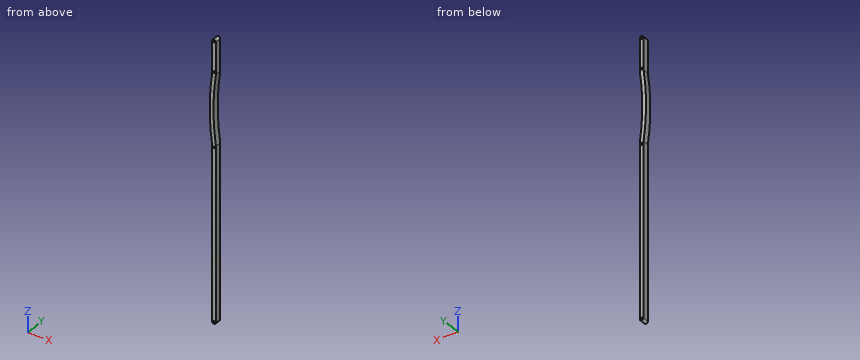
Autodesk Inventor part; units mm, degrees
ref_plane "YZ Plane" through (0, 0, 0) normal (1, 0, 0) x (0, 1, 0)
ref_plane "XZ Plane" through (0, 0, 0) normal (0, 1, 0) x (-1, 0, 0)
ref_plane "XY Plane" through (0, 0, 0) normal (0, 0, 1) x (1, 0, 0)
sketch "Sketch1" plane through (0, 0, 0) normal (0, 1, 0) x (-1, 0, 0)
  line L0 (0, 0) -> (0, -441.93) construction
  line L1 (-3, 0) -> (-3, -441.93)
  line L2 (3, -441.93) -> (3, 0)
  arc A0 (3, 0) -> (-3, 0) centre (0, 0) ccw
  arc A1 (-3, -441.93) -> (3, -441.93) centre (0, -441.93) ccw
  circle A2 centre (0, 0) radius 1.5
  circle A3 centre (0, -441.93) radius 1.5
  circle A4 centre (0, -48.203) radius 1.5
  circle A5 centre (0, -166.766) radius 1.5
  arc A6 (-3, -163.766) -> (-3, -51.203) centre (-399.0207, -107.4845) ccw
  arc A7 (3, -163.766) -> (3, -51.203) centre (-393.0207, -107.4845) ccw
  point P0 (0, -220.965)
  dimension "d0" = 6
  dimension "d1" = 441.93
  dimension "d2" = 3
  dimension "d3" = 3
  dimension "d20" = 3
  dimension "d21" = 48.203
  dimension "d22" = 3
  dimension "d23" = 166.766
  dimension "d24" = 400
  dimension "d25" = 400
  dimension "d26" = 3
  dimension "d28" = 3
extrude "Extrusion1" add sketch "Sketch1" along normal blind 10 contours A0 L2 A1 L1 A6 | A7 L2
sketch "Sketch2" plane through (0, 10, 0) normal (0, 1, 0) x (1, 0, 0)
  line L0 (3, 0) -> (3, 51.203)
  arc A0 (3, 163.766) -> (3, 51.203) centre (399.0207, 107.4845) ccw
  line L1 (3, 163.766) -> (3, 441.93)
  arc A1 (3, 441.93) -> (-3, 441.93) centre (0, 441.93) ccw
  line L2 (-3, 441.93) -> (-3, 163.766)
  arc A2 (-3, 163.766) -> (-3, 51.203) centre (393.0207, 107.4845) ccw
  line L3 (-3, 51.203) -> (-3, 0)
  arc A3 (-3, 0) -> (3, 0) centre (0, 0) ccw
  circle A4 centre (0, 0) radius 1.5
  circle A5 centre (0, 441.93) radius 1.5
  circle A6 centre (0, 166.766) radius 1.5
  circle A7 centre (0, 48.203) radius 1.5
  line L4 (-3, 258.3394) -> (0, 251.9059)
  line L5 (0, 251.9059) -> (3, 258.3394)
  dimension "d29" = 25
  dimension "d30" = 25
extrude "Extrusion2" [suppressed]
Design review of the part built by this model. Coordinates are the model's own, in mm. Give positions to 0.01 mm unless a question says otherwise; leave off trailing zeros. Order: outer loops, then holes, each group sorted by start corner. A loop starts at its lowest first (then second) coordinate and runs counter-clockwise, first axis right, second up. Notation, with made-up numbers: (-7.5, 35) -> (44.5, 35) arc R25 cw to (44.5, 48) -> close; hole circle Ø1 at (50.25, 15.25). An arc over 180 degrees is marked (long way). Write item = value, one per line. Start each with the question number.
(1) To check wall thickness, follow line 1 along X through (y, z) = (9, -321); line 2 along X through (y, z) = (5.75, -441.93); line 3 along Z through (x, y) = (-2.25, 3.5). State the ranges of each line that lie inside material, in increasing order.
(2) We need section A-A on y = 6.25. Write out the cut boundary in (x, z), plus the area to 3 significant figures.
(3) For pin 1 (3 mm diameter, centred on y = 5, z = -24, fed in from -X); pin 2 (1 mm diameter, centred on x = -4, z = -395.5, fed in from -Y), all flat-tipped, find the tip position at first contact; note any pin that passes through.
(4) We need section B-B on z = -255.5. Write out the cut boundary in (x, y).
Numbers:
q1.line_1 = -3 to 3
q1.line_2 = -3 to -1.5, 1.5 to 3
q1.line_3 = -443.91 to 1.98
q2.outline = (-3, -441.93) arc R3 ccw to (3, -441.93) -> (3, -163.77) arc R400 cw to (3, -51.2) -> (3, 0) arc R3 ccw to (-3, 0) -> (-3, -51.2) arc R400 ccw to (-3, -163.77) -> close; hole circle Ø3 at (0, -441.93); hole circle Ø3 at (0, -166.77); hole circle Ø3 at (0, -48.2); hole circle Ø3 at (0, 0)
q2.area = 2,650 mm^2
q3.pin_1 = -3
q3.pin_2 = through
q4.outline = (-3, 0) -> (3, 0) -> (3, 10) -> (-3, 10) -> close
